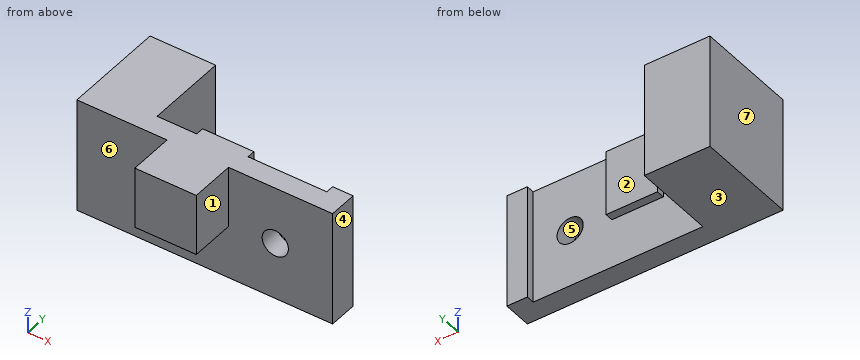
```python
from build123d import *

# Parameters (mm, degrees)
SKETCH_1_W         = 31.2
SKETCH_1_H         = 14
EXTRUDE_1_DEPTH    = 2.5
SKETCH_2_W         = 8
SKETCH_2_H         = 14
EXTRUDE_2_DEPTH    = 10
SKETCH_3_W         = 7.5
SKETCH_3_H         = 7.5
EXTRUDE_3_DEPTH    = 5.5
HOLE_WIZARD_M3_1_D = 3.2
SKETCH_9_W         = 6.266652583
SKETCH_9_H         = 7.99110138
EXTRUDE_7_DEPTH    = 1
SKETCH_10_W        = 2.5
SKETCH_10_H        = 14
EXTRUDE_8_DEPTH    = 1


with BuildPart() as part:
    # 草图1 → 凸台-拉伸1 (new body)
    with BuildSketch(Plane(origin=(0, 0, 0), x_dir=(1, 0, 0), z_dir=(0, 1, 0))):
        Rectangle(SKETCH_1_W, SKETCH_1_H)
    extrude(amount=EXTRUDE_1_DEPTH)

    # 草图2 → 凸台-拉伸2 (add)
    with BuildSketch(Plane(origin=(0, 2.5, 0), x_dir=(1, 0, 0), z_dir=(0, 1, 0))):
        with Locations((-11.6, 0)):
            Rectangle(SKETCH_2_W, SKETCH_2_H)
    extrude(amount=EXTRUDE_2_DEPTH)

    # 草图3 → 凸台-拉伸3 (add)
    with BuildSketch(Plane.XZ):
        with Locations((-0.85, 3.25)):
            Rectangle(SKETCH_3_W, SKETCH_3_H)
    extrude(amount=EXTRUDE_3_DEPTH)

    # M3 间隙孔1 (through all)
    with Locations(Plane(origin=(0, 2.5, 0), x_dir=(1, 0, 0), z_dir=(0, 1, 0))):
        with Locations((8.6, 0)):
            Hole(HOLE_WIZARD_M3_1_D / 2)

    # 草图9 → 凸台-拉伸7 (add)
    with BuildSketch(Plane(origin=(0, 2.5, 0), x_dir=(1, 0, 0), z_dir=(0, 1, 0))):
        with Locations((0.366673708, -3.00444931)):
            Rectangle(SKETCH_9_W, SKETCH_9_H)
    extrude(amount=EXTRUDE_7_DEPTH)

    # 草图10 → 凸台-拉伸8 (add)
    with BuildSketch(Plane.XZ.offset(-2.5)):
        with Locations((14.35, 0)):
            Rectangle(SKETCH_10_W, SKETCH_10_H)
    extrude(amount=-EXTRUDE_8_DEPTH)


solid = part.part
```
For this review, take the finished solid that the model builds, in its own axes (mm). Face numbers are marked on the shaded views. A direction names the side the tool comes from. Coordinates: 2 decimals unless noted, no trailing zeros. Order: outer loops, then holes, each group sorted by start corner. A loop starts at its lowest first (then second) coordinate and runs counter-clockwise, first axis right, second up. Notation, with made-up numbers: (-26.75, -31) -> (26.25, -31) arc R35 cw to (26.25, 4) -> close; hole circle Ø9 at (58.25, 73). An arc over 180 degrees is marked (long way). Answer as CSV lines item,"result".
Q1. Clearance check with flat-ended pins moving along their axes: pin 1 Ø2 at (x, z) = (14, -3) entering from +Y; pin 2 Ø6 at (y, z) = (-4, 3) entering from +X; pin 3 Ø5 at (x, z) = (8.6, 0) entering from -Y; pin 4 Ø3 at (y, z) = (-0.5, 2) entering from +X. State where each tip first meets the part, or that it passes through.
Model answer:
pin 1,"stops at y = 3.5"
pin 2,"stops at x = 2.9"
pin 3,"stops at y = 0"
pin 4,"stops at x = 15.6"
Q2. We need section C-C (x = -1.5). State the section outline as (y, z) points.
Model answer:
outline,"(-5.5, -0.5) -> (0, -0.5) -> (0, -7) -> (2.5, -7) -> (2.5, -0.99) -> (3.5, -0.99) -> (3.5, 7) -> (-5.5, 7) -> close"
Q3. We need section A-A (z = -3). State the section outline as (x, y) points, plus the area to 4 significant figures.
Model answer:
outline,"(-15.6, 0) -> (15.6, 0) -> (15.6, 3.5) -> (13.1, 3.5) -> (13.1, 2.5) -> (-7.6, 2.5) -> (-7.6, 12.5) -> (-15.6, 12.5) -> close"
area,"160.5 mm2"
Q4. Wall thickness on line 1 along Z through (x, y) = (8.6, 1.9); line 2 along X through (y, z) = (6.5, -1.25); line 3 along Y through (x, z) = (8, 3): over which ranges is each line inside the solid? List them lowest first. Write a range as [from, to].
Model answer:
line 1,"z = [-7, -1.6], [1.6, 7]"
line 2,"x = [-15.6, -7.6]"
line 3,"y = [0, 2.5]"
Q5. For the marked faces 1, 2 and 3, list the 3-axis set-ups (+Z, -Z, +X, -X, +Y, -Y) from which the entire face can be reached by the end or side of a thin tool; tool diameter is ignored.
Model answer:
face 1,"+Z, -Z, +X, -Y"
face 2,"+Z, -Z, +X, +Y"
face 3,"-Z, +X, -X, +Y, -Y"
Q6. Draft analysis for pull direction X (two halves, no side actions). For the marked faces 4, 5, 6 and 7, state which applies: released by +X, released by -X, zero draft, split by the parting line, or undercut.
Model answer:
face 4,"released by +X"
face 5,"undercut"
face 6,"zero draft"
face 7,"released by -X"
Q7. We need section B-B (x = 8.6). State the section outline as (y, z) points.
Model answer:
outline,"(0, -7) -> (2.5, -7) -> (2.5, -1.6) -> (0, -1.6) -> close; (0, 1.6) -> (2.5, 1.6) -> (2.5, 7) -> (0, 7) -> close"
Q8. We need section D-D (z = 0). State the section outline as (x, y) points.
Model answer:
outline,"(-15.6, 0) -> (-4.6, 0) -> (-4.6, -5.5) -> (2.9, -5.5) -> (2.9, 0) -> (7, 0) -> (7, 2.5) -> (3.5, 2.5) -> (3.5, 3.5) -> (-2.77, 3.5) -> (-2.77, 2.5) -> (-7.6, 2.5) -> (-7.6, 12.5) -> (-15.6, 12.5) -> close; (10.2, 0) -> (15.6, 0) -> (15.6, 3.5) -> (13.1, 3.5) -> (13.1, 2.5) -> (10.2, 2.5) -> close"
